Design review of the part built by this model. Coordinates are the model's own, in mm. A direction names the side the tool comes from. Round coordinates to 2 decimals unless told otherwise and drop trailing zeros. Write each loop counter-clockwise with the first axis right and the second up, starting at its lowest first coordinate (ties: lowest second). Pieces come first, ordered by that corner, then holes. Notation, with made-up numbers: (-16.5, 81.25) -> (-7.5, 81.25) arc R5 cw to (-7.5, 89.25) -> close; hole circle Ø3 at (-23.75, 54). An arc over 180 degrees is marked (long way). Write item = value, one per line. Start each with the question number.
Item 1: Add section C-C, the plane z = -17.5. State how many separate pieces and enclosed holes the cut face has, then the cut area to 3 significant figures.
Item 2: Machinability: for faces 4 (the flat face through (-56.897, -1, -1)), 5 (the cylindrical face through (71.51, 0.8, -68.04)), 6 (the cylindrical face through (63.158, -12.613, -54.645)), 7 (the cylindrical face through (-0.8, -71.41, 67.94)), which of the approach directions +Z, -Z, +X, -X, +Y, -Y give a long, thin tool a straight path to every point of the face, cutting with its end or side? Answer none if there is none.
Item 3: To check wall thickness, follow L1, parallel to Z at x = 45.5, y = 88; L2, parallel to Y at x = 7, z = 59. State the ranges of each line that lie inside material, in increasing order.
Item 4: Mouldability with a two-part tool opening along Y and no side actions: class faces 1 (the cylindrical face through (0.8, -71.51, -68.04)), 2 (the cylindrical face through (50.11, 81.425, 76.289)), 3 (the flat face through (7, 77, -69.85)) as released by +Y, released by -Y, zero draft, split by the parting line, or undercut.
Item 5: Add section B-B, the plane x = -8. State the section outline as (y, z) points, then the cut area to 3 significant figures.
Item 6: For pin 1 Ø15 at (y, z) = (19.05, 47.625) entering from -X; pin 2 Ø22 at (y, z) = (-19.05, -47.625) entering from -X; pin 3 Ø25 at (y, z) = (19.05, 15.875) entering from +X; pin 4 Ø12 at (x, z) = (-67, -60) entering from -Y, all flat-tipped, find the tip position at first contact; note any pin that passes through.
Item 7: Add section A-A, the plane z = 30. State the section outline as (x, y) points.
from build123d import *

# Parameters (mm, degrees)
SKETCH2_W               = 139.193969876
SKETCH2_H               = 139.193969876
BOSS_EXTRUDE1_DEPTH     = 76.2
SKETCH3_R               = 104.775
BOSS_EXTRUDE2_DEPTH     = 6.35
SKETCH4_R               = 104.775
BOSS_EXTRUDE3_DEPTH     = 6.35
CUT_EXTRUDE1_DEPTH      = 170.617521943
CUT_EXTRUDE1_DEPTH_BACK = 170.617521943
SKETCH2_3_W             = 113.793969876
SKETCH2_3_H             = 113.793969876
FILLET1_R               = 12.7
SKETCH6_R               = 3.18262
CUT_EXTRUDE2_DEPTH      = 222.841410133
CIRPATTERN1_COUNT       = 12
SKETCH8_R               = 9.525
CUT_EXTRUDE3_DEPTH      = 220.540183694
FILLET2_R               = 6.35


with BuildPart() as part:
    # Sketch2 → Boss-Extrude1 (new, symmetric)
    with BuildSketch(Plane.XY):
        Rectangle(SKETCH2_W, SKETCH2_H)
    extrude(amount=BOSS_EXTRUDE1_DEPTH, both=True)

    # Sketch3 → Boss-Extrude2 (add, symmetric)
    with BuildSketch(Plane.XY.offset(76.2)):
        Circle(SKETCH3_R)
    extrude(amount=BOSS_EXTRUDE2_DEPTH, both=True)

    # Sketch4 → Boss-Extrude3 (add, symmetric)
    with BuildSketch(Plane(origin=(0, 0, -76.2), x_dir=(-1, 0, 0), z_dir=(0, 0, -1))):
        with Locations(Location((0, 0, 0), (0, 0, 180))):
            Circle(SKETCH4_R)
    extrude(amount=BOSS_EXTRUDE3_DEPTH, both=True)

    # Sketch2_3 → Cut-Extrude1 (cut, two sides: drawn at the far end of the back side and taken through both)
    with BuildSketch(Plane.XY.offset(-CUT_EXTRUDE1_DEPTH_BACK)):
        Rectangle(SKETCH2_3_W, SKETCH2_3_H)
    extrude(amount=CUT_EXTRUDE1_DEPTH + CUT_EXTRUDE1_DEPTH_BACK, mode=Mode.SUBTRACT)

    # Fillet1
    fillet1_edges = [part.edges().sort_by_distance(p)[0] for p in [
        (-69.596984938, 69.596984938, 0),
        (69.596984938, 69.596984938, 0),
        (69.596984938, -69.596984938, 0),
        (-69.596984938, -69.596984938, 0),
        (-56.896984938, -56.896984938, 0),
        (-56.896984938, 56.896984938, 0),
        (56.896984938, 56.896984938, 0),
        (56.896984938, -56.896984938, 0),
    ]]
    fillet(fillet1_edges, radius=FILLET1_R)

    # Sketch6 → Cut-Extrude2 (cut, symmetric)
    with BuildSketch(Plane.XY.offset(82.55)):
        with Locations((48.641, 84.248683331)):
            Circle(SKETCH6_R)
    cut_extrude2 = extrude(amount=CUT_EXTRUDE2_DEPTH, both=True, mode=Mode.SUBTRACT)

    # CirPattern1: Cut-Extrude2 ×12 about axis
    cirpattern1_axis = Axis((0, 0, 0), (0, 0, 1))
    for i in range(1, CIRPATTERN1_COUNT):
        add(cut_extrude2.rotate(cirpattern1_axis, i * 360 / CIRPATTERN1_COUNT), mode=Mode.SUBTRACT)

    # Sketch8 → Cut-Extrude3 (cut, through all)
    with BuildSketch(Plane.ZY.offset(69.596984938)):
        with Locations((-47.625, 19.05)):
            Circle(SKETCH8_R)
        with Locations((47.625, 19.05)):
            Circle(SKETCH8_R)
        with Locations((-15.875, 19.05)):
            Circle(SKETCH8_R)
        with Locations((15.875, 19.05)):
            Circle(SKETCH8_R)
        with Locations((15.875, -19.05)):
            Circle(SKETCH8_R)
        with Locations((-15.875, -19.05)):
            Circle(SKETCH8_R)
        with Locations((47.625, -19.05)):
            Circle(SKETCH8_R)
        with Locations((-47.625, -19.05)):
            Circle(SKETCH8_R)
    extrude(amount=-CUT_EXTRUDE3_DEPTH, mode=Mode.SUBTRACT)

    # Fillet2
    fillet2_edges = [part.edges().sort_by_distance(p)[0] for p in [
        (69.596984938, 0, -69.85),
        (69.596984938, 0, 69.85),
        (0, -69.596984938, -69.85),
        (0, -69.596984938, 69.85),
        (-69.596984938, 0, -69.85),
        (-69.596984938, 0, 69.85),
        (0, 69.596984938, -69.85),
        (0, 69.596984938, 69.85),
        (65.877241059, -65.877241059, -69.85),
        (65.877241059, -65.877241059, 69.85),
        (-65.877241059, -65.877241059, -69.85),
        (-65.877241059, -65.877241059, 69.85),
        (65.877241059, 65.877241059, -69.85),
        (65.877241059, 65.877241059, 69.85),
        (-65.877241059, 65.877241059, -69.85),
        (-65.877241059, 65.877241059, 69.85),
    ]]
    fillet(fillet2_edges, radius=FILLET2_R)


solid = part.part
Result set:
q1.separate_pieces = 4
q1.enclosed_holes = 0
q1.area = 5,470 mm²
q2.face_4 = +Z, -Z
q2.face_5 = +X, +Y, -Y
q2.face_6 = +X, -X
q2.face_7 = +X, -X, -Y
q3.L1 = -82.55 to -69.85, 69.85 to 82.55
q3.L2 = -69.6 to -56.9, 56.9 to 69.6
q4.face_1 = released by -Y
q4.face_2 = undercut
q4.face_3 = zero draft
q5.outline = (-104.47, -82.55) -> (-56.9, -82.55) -> (-56.9, 82.55) -> (-104.47, 82.55) -> (-104.47, 69.85) -> (-75.95, 69.85) arc R6.35 cw to (-69.6, 63.5) -> (-69.6, -63.5) arc R6.35 cw to (-75.95, -69.85) -> (-104.47, -69.85) -> close; (56.9, -82.55) -> (104.47, -82.55) -> (104.47, -69.85) -> (75.95, -69.85) arc R6.35 cw to (69.6, -63.5) -> (69.6, 63.5) arc R6.35 cw to (75.95, 69.85) -> (104.47, 69.85) -> (104.47, 82.55) -> (56.9, 82.55) -> close
q5.area = 6,000 mm²
q6.pin_1 = through
q6.pin_2 = -69.6
q6.pin_3 = 69.6
q6.pin_4 = -68.92
q7.outline = (-69.6, -56.9) arc R12.7 ccw to (-56.9, -69.6) -> (56.9, -69.6) arc R12.7 ccw to (69.6, -56.9) -> (69.6, 56.9) arc R12.7 ccw to (56.9, 69.6) -> (-56.9, 69.6) arc R12.7 ccw to (-69.6, 56.9) -> close; hole (-56.9, -44.2) arc R12.7 ccw to (-44.2, -56.9) -> (44.2, -56.9) arc R12.7 ccw to (56.9, -44.2) -> (56.9, 44.2) arc R12.7 ccw to (44.2, 56.9) -> (-44.2, 56.9) arc R12.7 ccw to (-56.9, 44.2) -> close
